```python
from build123d import *

# Parameters (mm, degrees)
SKICA1_R        = 3
VYSUNOUT1_DEPTH = 20


with BuildPart() as part:
    # Skica1 → Vysunout1 (new, symmetric)
    with BuildSketch(Plane.XY):
        Circle(SKICA1_R)
    extrude(amount=VYSUNOUT1_DEPTH, both=True)

    # Skica2 → Díra1 (revolve, cut)
    with BuildSketch(Plane(origin=(0, 0, 20), x_dir=(0, -1, 0), z_dir=(1, 0, 0))):
        Polygon((0, 0), (0, 5.201721238), (2, 4), (2, 0), align=None)
    d_ra1 = revolve(axis=Axis((0, 0, 24.244199587), (0, 0, -1)), mode=Mode.SUBTRACT)

    # Zrcadlit1: Díra1 across plane
    add(d_ra1.mirror(Plane.XY), mode=Mode.SUBTRACT)


solid = part.part
```
Here's how the part is built. I have some questions about the finished solid (model axes, mm). A direction names the side the tool comes from. Coordinates: 2 decimals unless noted, no trailing zeros. Loops run counter-clockwise (first coordinate to the right, second up) from the corner with the lowest first, then second, coordinate; pieces in that order, holes last. Notation, with made-up numbers: (-9, 8.25) -> (6, 8.25) arc R11 cw to (6, 29.25) -> close; hole circle Ø3 at (6.5, 62). An arc over 180 degrees is marked (long way). Return JSON: item names as keys, results as strings.
1) If we section it at B-B, the plane z = -12: Write out the boundary of the cut face in (x, y), then the cut area to 3 significant figures.
Results below:
{"outline": "circle Ø6 at (0, 0)", "area": "28.3 mm²"}
2) I need wall thicknesses on line 1 (Y direction, x = 0, z = 17.05); line 2 (Y direction, x = -0.5, z = 17); line 3 (X direction, y = -0.1, z = -15). Which ranges of each line are inside material? Lowest first, please. Write a range as from..to.
Results below:
{"line 1": "-3..-2, 2..3", "line 2": "-2.96..-1.94, 1.94..2.96", "line 3": "-3..-0.32, 0.32..3"}
3) For faces 4 (the face through (2, 0, -18)), 5 (the face through (0.34, 0.08, 15.01)), which set-ups out of +Z, -Z, +X, -X, +Y, -Y let a thin tool reach every point of the face, with its end or its side?
Results below:
{"face 4": "-Z", "face 5": "+Z"}
4) Thinking about a two-plate mould opening in X: for faces 1 (the face through (1, -2, 20)), 2 (the face through (2, 0, 18)), 3 (the face through (-3, 0, 0)), which applies, +X half, -X half, draft (parallel to the pull), parting line (faces both ways), or undercut?
Results below:
{"face 1": "draft", "face 2": "undercut", "face 3": "parting line"}
5) Will these pins go through, and if not, where does the flat tip stop? pin 1 (3 mm diameter, centred on x = -2, z = -10, fed in from -Y); pin 2 (3 mm diameter, centred on x = 0, y = 0, fed in from -Z); pin 3 (1.5 mm diameter, centred on x = -2.5, z = -13, fed in from +Y).
Results below:
{"pin 1": "y = -2.96", "pin 2": "z = -15.7", "pin 3": "y = 2.44"}
6) If we section it at A-A, the plane z = 17: Write out the boundary of the cut face in (x, y), then the cut area to 3 significant figures.
Results below:
{"outline": "circle Ø6 at (0, 0); hole circle Ø4 at (0, 0)", "area": "15.7 mm²"}
